Geometry check sheet. Reference: the model listing, model coordinates, mm. Face numbers are marked on the shaded views. A direction names the side the tool comes from. Round coordinates to 2 decimals unless told otherwise and drop trailing zeros. Order: outer loops, then holes, each group sorted by start corner. A loop starts at its lowest first (then second) coordinate and runs counter-clockwise, first axis right, second up. Notation, with made-up numbers: (73, 64) - (97, 64) arc R6 ccw to (97, 68) - close; hole circle Ø8 at (-19, 25). An arc over 180 degrees is marked (long way). Answer as CSV lines item,"result". Start each with the question number.
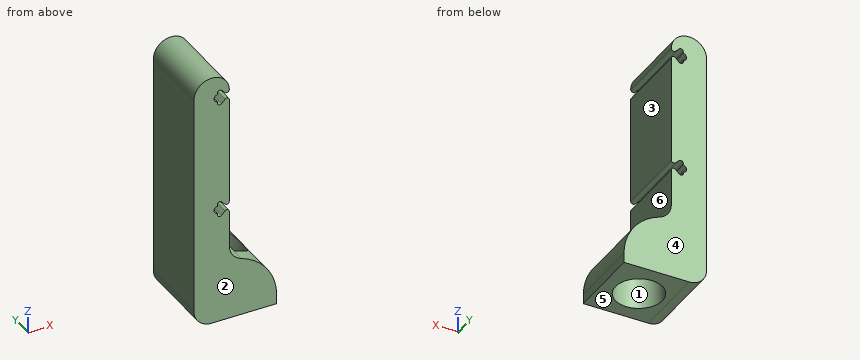
```python
from build123d import *

# Parameters (mm, degrees)
BOSS_EXTRUDE1_DEPTH = 12.7
SKETCH2_R           = 4
CUT_EXTRUDE1_DEPTH  = 10


with BuildPart() as part:
    # Sketch1 → Boss-Extrude1 (new body)
    with BuildSketch(Plane(origin=(0, 0, 0), x_dir=(1, 0, 0), z_dir=(0, 1, 0))):
        with BuildLine():
            Line((-4.055343897, 0.632583633), (-4.075844459, 0.866906139))
            ThreePointArc((-4.075844459, 0.866906139), (-3.83530083, 1.283539926), (-3.361522369, 1.2))
            Line((-3.361522369, 1.2), (-2.761522369, 0.6))
            ThreePointArc((-2.761522369, 0.6), (-2.304491577, 0.509090923), (-2.04560443, 0.89654292))
            Line((-2.04560443, 0.89654292), (-2.04560443, 19.10345708))
            ThreePointArc((-2.04560443, 19.10345708), (-2.304491577, 19.490909077), (-2.761522369, 19.4))
            Line((-2.761522369, 19.4), (-3.361522369, 18.8))
            ThreePointArc((-3.361522369, 18.8), (-3.83530083, 18.716460074), (-4.075844459, 19.133093861))
            Line((-4.075844459, 19.133093861), (-4.055343897, 19.367416367))
            ThreePointArc((-4.055343897, 19.367416367), (-4.635, 20), (-4.055343897, 20.632583633))
            Line((-4.055343897, 20.632583633), (-4.075844459, 20.866906139))
            ThreePointArc((-4.075844459, 20.866906139), (-3.83530083, 21.283539926), (-3.361522369, 21.2))
            Line((-3.361522369, 21.2), (-2.761522369, 20.6))
            ThreePointArc((-2.761522369, 20.6), (-2.304491577, 20.509090923), (-2.04560443, 20.89654292))
            Line((-2.04560443, 20.89654292), (-2.04560443, 27.15586057))
            ThreePointArc((-2.04560443, 27.15586057), (-1.481090696, 28.90754737), (0, 30))
            ThreePointArc((0, 30), (4.34421438, 33.204292914), (6, 38.342197704))
            Line((6, 38.342197704), (6, 40))
            Line((6, 40), (-5.04560443, 40))
            ThreePointArc((-5.04560443, 40), (-7.166924773, 39.121320344), (-8.04560443, 37))
            Line((-8.04560443, 37), (-8.04560443, -0.89654292))
            ThreePointArc((-8.04560443, -0.89654292), (-5.04560443, -3.89654292), (-2.04560443, -0.89654292))
            ThreePointArc((-2.04560443, -0.89654292), (-2.304491577, -0.509090923), (-2.761522369, -0.6))
            Line((-2.761522369, -0.6), (-3.361522369, -1.2))
            ThreePointArc((-3.361522369, -1.2), (-3.83530083, -1.283539926), (-4.075844459, -0.866906139))
            Line((-4.075844459, -0.866906139), (-4.055343897, -0.632583633))
            ThreePointArc((-4.055343897, -0.632583633), (-4.635, 0), (-4.055343897, 0.632583633))
        make_face()
    extrude(amount=BOSS_EXTRUDE1_DEPTH)

    # Sketch2 → Cut-Extrude1 (cut)
    with BuildSketch(Plane(origin=(0, 0, -40), x_dir=(-1, 0, 0), z_dir=(0, 0, -1))):
        with Locations((0, 6.35)):
            Circle(SKETCH2_R)
    extrude(amount=-CUT_EXTRUDE1_DEPTH, mode=Mode.SUBTRACT)


solid = part.part
```
1. Thickness scan on probe 1 along Y at (x, z) = (0, -31.75); probe 2 along Z at (x, y) = (-4, 2.25); probe 3 along Z at (x, y) = (-3.5, 3.5). Record the ranges inside material, lowest first.
2. Section check D-D on z = -34.5. Record the boundary of the cut face in (x, y).
3. Access from +Z, -Z, +X, -X, +Y, -Y to the whole of each face (thin tool, end or side, straight path). Record for the marked faces 5 and 6.
4. Section check A-A on x = 2.75. Record the boundary of the cut face in (y, z), plus the area to 3 significant figures.
5. Draft check along Y on the marked faces 1, 2, 3 and 4. Enter one of: released by +Y, released by -Y, zero draft, split by the parting line, or undercut.
6. Section check C-C on y = 11.25. Record the boundary of the cut face in (x, z) (3 decimals), plus the area to 3 significant figures.
7. Go/stop test with flat-tipped pins: pin 1 Ø6 at (x, y) = (-2, 6.5) entering from -Z; pin 2 Ø3 at (y, z) = (8, -23) entering from +X; pin 3 Ø3 at (y, z) = (10, -33) entering from +X. Record where each tip stops, or that it passes through.
Numbers:
1,probe 1,"y = 0 to 2.35, 10.35 to 12.7"
1,probe 2,"z = -40 to -21.15, -18.85 to -1.15, 1.15 to 3.71"
1,probe 3,"z = -40 to -21.29, -18.71 to -1.29, 1.29 to 3.47"
2,outline,"(-8.05, 0) - (5.12, 0) - (5.12, 12.7) - (-8.05, 12.7) - close; hole circle Ø8 at (0, 6.35)"
3,face 5,"-Z, +X, -X, +Y, -Y"
3,face 6,"+Z, +X, +Y, -Y"
4,outline,"(0, -40) - (3.45, -40) - (3.45, -31.51) - (0, -31.51) - close; (9.25, -40) - (12.7, -40) - (12.7, -31.51) - (9.25, -31.51) - close"
4,area,"58.5 mm2"
5,face 1,"undercut"
5,face 2,"released by -Y"
5,face 3,"zero draft"
5,face 4,"released by +Y"
6,outline,"(-8.046, -37) arc R3 ccw to (-5.046, -40) - (6, -40) - (6, -38.342) arc R8.799 ccw to (0, -30) arc R3 cw to (-2.046, -27.156) - (-2.046, -20.897) arc R0.419 ccw to (-2.762, -20.6) - (-3.362, -21.2) arc R0.419 cw to (-4.076, -20.867) - (-4.055, -20.633) arc R0.635 cw to (-4.055, -19.367) - (-4.076, -19.133) arc R0.419 cw to (-3.362, -18.8) - (-2.762, -19.4) arc R0.419 ccw to (-2.046, -19.103) - (-2.046, -0.897) arc R0.419 ccw to (-2.762, -0.6) - (-3.362, -1.2) arc R0.419 cw to (-4.076, -0.867) - (-4.055, -0.633) arc R0.635 cw to (-4.055, 0.633) - (-4.076, 0.867) arc R0.419 cw to (-3.362, 1.2) - (-2.762, 0.6) arc R0.419 ccw to (-2.046, 0.897) arc R3 ccw to (-8.046, 0.897) - close"
6,area,"318 mm2"
7,pin 1,"stops at z = -40"
7,pin 2,"stops at x = -2.05"
7,pin 3,"stops at x = 5.12"
